Input: part model. Units: mm. Frame: model coordinates. Round coordinates to 2 decimals unless told otherwise and drop trailing zeros. Order: outer loops, then holes, each group sorted by start corner. A loop starts at its lowest first (then second) coordinate and runs counter-clockwise, first axis right, second up. Notation, with made-up numbers: M 84,36 L 101,36 A22 cw 101,53 Z; hole C 50.5,42.5 d4. An arc over 180 degrees is marked long. One line per question, with ' | ' between items.
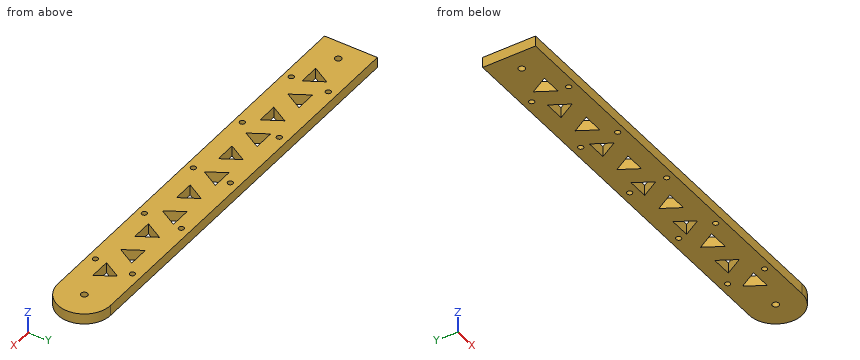
Autodesk Inventor part; units mm, degrees
ref_plane "YZ Plane" through (0, 0, 0) normal (1, 0, 0) x (0, 1, 0)
ref_plane "XZ Plane" through (0, 0, 0) normal (0, 1, 0) x (-1, 0, 0)
ref_plane "XY Plane" through (0, 0, 0) normal (0, 0, 1) x (1, 0, 0)
sketch "Sketch1" plane through (0, 0, 0) normal (0, 0, 1) x (1, 0, 0)
  line L0 (0, 0) -> (484.886, 0)
  line L1 (484.886, 63.5) -> (0, 63.5)
  line L2 (0, 63.5) -> (0, 0)
  circle A0 centre (73.914, 53.3905) radius 3.175
  circle A1 centre (162.9664, 53.3905) radius 3.175
  circle A2 centre (252.0188, 53.3868) radius 3.175
  circle A3 centre (341.0712, 53.3868) radius 3.175
  circle A4 centre (430.1236, 53.3868) radius 3.175
  circle A5 centre (73.914, 8.9405) radius 3.175
  circle A6 centre (162.9664, 8.9368) radius 3.175
  circle A7 centre (252.0188, 8.9368) radius 3.175
  circle A8 centre (341.0712, 8.9368) radius 3.175
  circle A9 centre (430.1236, 8.9368) radius 3.175
  line L3 (61.214, 43.0781) -> (73.5873, 21.6469)
  line L4 (48.8407, 21.6469) -> (61.214, 43.0781)
  line L5 (137.414, 43.0781) -> (149.7873, 21.6469)
  line L6 (149.7873, 21.6469) -> (125.0407, 21.6469)
  line L7 (125.0407, 21.6469) -> (137.414, 43.0781)
  line L8 (99.314, 21.6469) -> (86.9407, 43.0781)
  line L9 (86.9407, 43.0781) -> (111.6873, 43.0781)
  line L10 (111.6873, 43.0781) -> (99.314, 21.6469)
  line L11 (48.8407, 21.6469) -> (73.5873, 21.6469)
  line L12 (289.4838, 43.0781) -> (301.8571, 21.6469)
  line L13 (301.8571, 21.6469) -> (277.1105, 21.6469)
  line L14 (277.1105, 21.6469) -> (289.4838, 43.0781)
  line L15 (263.7571, 43.0781) -> (251.3838, 21.6469)
  line L16 (251.3838, 21.6469) -> (239.0105, 43.0781)
  line L17 (239.0105, 43.0781) -> (263.7571, 43.0781)
  line L18 (213.2838, 43.0781) -> (225.6571, 21.6469)
  line L19 (200.9105, 21.6469) -> (225.6571, 21.6469)
  line L20 (200.9105, 21.6469) -> (213.2838, 43.0781)
  line L21 (441.5536, 43.0781) -> (453.9269, 21.6469)
  line L22 (453.9269, 21.6469) -> (429.1803, 21.6469)
  line L23 (429.1803, 21.6469) -> (441.5536, 43.0781)
  line L24 (415.8269, 43.0781) -> (403.4536, 21.6469)
  line L25 (403.4536, 21.6469) -> (391.0803, 43.0781)
  line L26 (391.0803, 43.0781) -> (415.8269, 43.0781)
  line L27 (365.3536, 43.0781) -> (377.7269, 21.6469)
  line L28 (352.9803, 21.6469) -> (377.7269, 21.6469)
  line L29 (352.9803, 21.6469) -> (365.3536, 43.0781)
  line L30 (175.5175, 21.6469) -> (163.1442, 43.0781)
  line L31 (163.1442, 43.0781) -> (187.8909, 43.0781)
  line L32 (187.8909, 43.0781) -> (175.5175, 21.6469)
  line L33 (339.9607, 43.0781) -> (327.5873, 21.6469)
  line L34 (327.5873, 21.6469) -> (315.214, 43.0781)
  line L35 (315.214, 43.0781) -> (339.9607, 43.0781)
  line L36 (15.7817, 31.75) -> (30.4463, 31.75)
  circle A10 centre (23.114, 31.75) radius 4.0005
  circle A11 centre (484.886, 31.75) radius 4.0005
  arc A12 (484.886, 0) -> (484.886, 63.5) centre (484.886, 31.75) ccw
  point P0 (135.1884, 47.8306)
  point P1 (135.1884, 33.5431)
  point P2 (23.114, 19.05)
  point P3 (23.114, 25.4)
  point P4 (287.2582, 33.5431)
  point P5 (439.328, 33.5431)
  dimension "d18" = 44.45
  dimension "d36" = 56.5658
  dimension "d69" = 126.3396
  dimension "d72" = 25.4
  dimension "d12" = 6.35
  dimension "d15" = 89.0524
  dimension "d44" = 6.35
  dimension "d66" = 100.9467
  dimension "d97" = 152.0698
  dimension "d102" = 51.1231
  dimension "d115" = 8.001
extrude "Extrusion1" add sketch "Sketch1" along normal blind 12.7 contours L2 L1 A12 L0 | L3 L11 L4 | L12 L13 L14 | L15 L16 L17 | L18 L19 L20 | L21 L22 L23 | L24 L25 L26 | L27 L28 L29 | L30 L31 L32 | L33 L34 L35 | A10 L36 | L36 A10 | A11
extrude "Extrusion4" cut sketch "Sketch1" along normal blind 12.7 contours L3 L11 L4
extrude "Extrusion5" cut sketch "Sketch1" along normal blind 12.7 contours L12 L13 L14 | L15 L16 L17 | L18 L19 L20 | L21 L22 L23 | L24 L25 L26 | L27 L28 L29 | L30 L31 L32 | L33 L34 L35
extrude "Extrusion6" cut sketch "Sketch1" along normal blind 25.4 contours A11
extrude "Extrusion7" cut sketch "Sketch1" along normal blind 25.4 contours A10 L36 | L36 A10
properties part number "arm_plate_evan"
Item 1: Section query B-B, the plane z = 10.75. Give the number of separate pieces and of enclosed holes in the cut face, plus the area to 3 significant figures.
Report:
separate pieces: 1 | enclosed holes: 23 | area: 29,000 mm²
Item 2: Section query A-A, the plane x = 410.5. Return loops of the section in (y, z), plus the area to 3 significant figures.
Report:
outline: M 0,0 L 33.85,0 L 33.85,12.7 L 0,12.7 Z; M 43.08,0 L 63.5,0 L 63.5,12.7 L 43.08,12.7 Z | area: 689 mm²
Item 3: Line query: line 1 along X through (y, z) = (51, 4); line 2 along Y through (x, z) = (174.5, 7.25); line 3 along X through (y, z) = (10, 3.25). Output: solid intervals per line, ascending. Write a range as from..to.
Report:
line 1: 0..71.82, 76..160.88, 165.06..249.93, 254.11..338.98, 343.16..428.03, 432.22..510.13 | line 2: 0..23.41, 43.08..63.5 | line 3: 0..70.92, 76.91..159.97, 165.96..249.03, 255.01..338.08, 344.06..427.13, 433.12..508.02
